Input: dimensioned drawing with shaded views. Units: mm. Origin: part minimum x, y, z. A direction names the side the tool comes from. Coordinates: 2 decimals unless noted, no trailing zeros. Write each loop counter-clockwise with the first axis right and the second up, starting at its lowest first coordinate (ties: lowest second). Pieces come first, ordered by that corner, then holes. Notation, with made-up numbers: (-35.75, -30.5) -> (-9.75, -30.5) arc R34 cw to (-9.75, 8.5) -> close; hole circle Ø9 at (65.5, -24). An arc over 180 degrees is marked (long way). One line per item, written item: value. Start each with the question number.
1. Section query C-C, the plane y = 8.75. State how many separate pieces and enclosed holes the cut face has, and give its area (3 significant figures).
2. Section query A-A, the plane x = 17.5. Output: boundary loops of the cut face in (y, z), and give its area (3 significant figures).
3. Access query for the marked faces 1, 2 and 3. Directions: +Z, -Z, +X, -X, +Y, -Y. A direction counts if a zero-diameter tool reaches every point of the face in a straight line with its end or side. Return the directions, or none.
4. First-contact query: P1, Ø3.5, axis at x = 10, y = 10, coming from the +Z side; P2, Ø5, axis at x = 18, z = 10.5, coming from the +Y side; P3, Ø3, axis at y = 9.5, z = 9.5, coming from the +X side; P4, Ø4, axis at x = 17.5, y = 8, coming from the +Z side. Flat tips, straight axial feed; report the tip coordinate or a pass-through.
5. Line query: line 1 (Z direction, x = 17.5, y = 1.1); line 2 (Z direction, x = 16.5, y = 2.75); line 3 (X direction, y = 11, z = 7.5). Output: solid intervals per line, ascending.
6. Section query B-B, the plane z = 3.5. Output: boundary loops of the cut face in (x, y).
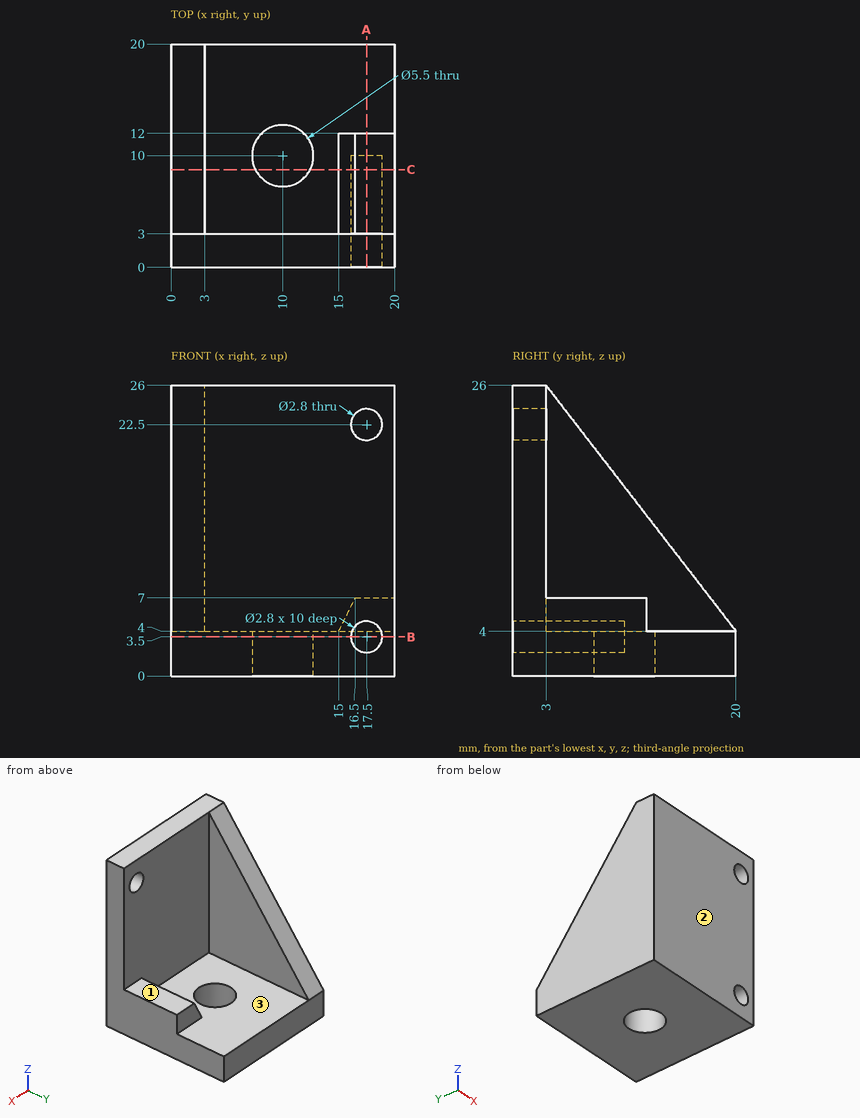
Computed values:
1. separate pieces: 2
1. enclosed holes: 1
1. area: 111 mm²
2. outline: (0, 0) -> (20, 0) -> (20, 4) -> (12, 4) -> (12, 7) -> (3, 7) -> (3, 21.1) -> (0, 21.1) -> (0, 4.9) -> (10, 4.9) -> (10, 2.1) -> (0, 2.1) -> close; (0, 23.9) -> (3, 23.9) -> (3, 26) -> (0, 26) -> close
2. area: 137 mm²
3. face 1: +Z, +X, +Y
3. face 2: +Z, -Z, +X, -X, -Y
3. face 3: +Z, +Y
4. P1: passes through
4. P2: stops at y = 3
4. P3: stops at x = 3
4. P4: stops at z = 7
5. line 1: z = 0 to 2.1, 4.9 to 21.1, 23.9 to 26
5. line 2: z = 0 to 2.52, 4.48 to 21.52, 23.48 to 26
5. line 3: x = 0 to 3
6. outline: (0, 0) -> (16.1, 0) -> (16.1, 10) -> (18.9, 10) -> (18.9, 0) -> (20, 0) -> (20, 20) -> (0, 20) -> close; hole circle Ø5.5 at (10, 10)
